```python
from build123d import *

# Parameters (mm, degrees)
F0_W        = 47.8297565132
F0_H        = 76.5759237111
F1_DEPTH    = 40
F2_T1_DEPTH = 274.1378594542
F3_T        = -2


# Not quite as in the source:
# - a fillet or chamfer that OpenCascade refuses, or shapes differently, is made with other operations: its cross-section is extruded or revolved along the edge and cut away or added


with BuildPart() as f1:
    # F0 (on Top) → F1 (new body)
    with BuildSketch(Plane.XY):
        with Locations((-40.5828235671, -10.7496175915)):
            Rectangle(F0_W, F0_H)
    extrude(amount=F1_DEPTH)

    # F2: chamfer of 44 on 1 edges, made by hand

    # F2_s2 → F2_t1 (cut)
    with BuildSketch(Plane.YZ.offset(-177.6517532942)):
        Polygon((27.538344264, -4), (-16.461655736, 40), (27.538344264, 40), align=None)
    extrude(amount=F2_T1_DEPTH, mode=Mode.SUBTRACT)

    # F3
    f3_openings = [f1.faces().sort_by_distance(p)[0] for p in [
        (-40.582824, 3.538344, 20),
    ]]
    offset(amount=F3_T, openings=f3_openings, kind=Kind.INTERSECTION)


solid = f1.part
```
The model under review builds one solid part; all positions refer to its coordinate system, in mm. A direction names the side the tool comes from. Coordinates: 2 decimals unless noted, no trailing zeros. Write each loop counter-clockwise with the first axis right and the second up, starting at its lowest first coordinate (ties: lowest second). Pieces come first, ordered by that corner, then holes. Notation, with made-up numbers: (-20, -25.75) - (-14, -25.75) arc R18 cw to (-14, -20.75) - close; hole circle Ø11 at (76, -25). An arc over 180 degrees is marked (long way). Answer in a Markdown table with one row per item. Add a question column.
Q1. Draft analysis for pull direction X (two halves, no side actions). For faces 3 (the face through (-16.668, -21, 15)), 4 (the face through (-41, -12, 2)), 5 (the face through (-41, -33, 40)), state which applies: +X half, -X half, draft (parallel to the pull), parting line (faces both ways), or undercut.
Q2. To check wall thickness, follow line 1 along X through (y, z) = (-32, 35); line 2 along Z through (x, y) = (-33, -34); line 3 along Y through (x, z) = (-39, 22.5). State the ranges of each line that lie inside material, in increasing order. Write a range as from..to.
Q3. Consider section B-B on y = 2. Give the boundary of the cut face in (x, z).
Q4. For faces 1 (the face through (-41, -47.038, 20)), 2 (the face through (-41, -49.038, 20)), list the 3-axis set-ups (+Z, -Z, +X, -X, +Y, -Y) from which the entire face can be reached by the end or side of a thin tool; tool diameter is ignored.
Q5. Clearance check with flat-ended pins moving along their axes: pin 1 (3 mm diameter, centred on x = -31, y = -7, fed in from +Z); pin 2 (6 mm diameter, centred on x = -31, z = 30, fed in from +Y); pin 3 (4 mm diameter, centred on x = -52, y = -14, fed in from +Z). State where each tip first meets the part, or that it passes through.
Q6. Consider section A-A on y = -30. Give the boundary of the cut face in (x, z).
Q7. Consider section C-C on x = -48. Give the boundary of the cut face in (y, z), then the cut area to 3 significant figures.
Answers below:
| question | item | result |
|---|---|---|
| 1 | face 3 | +X half |
| 1 | face 4 | undercut |
| 1 | face 5 | draft |
| 2 | line 1 | -64.5..-62.5, -18.67..-16.67 |
| 2 | line 2 | 0..2, 38..40 |
| 2 | line 3 | -49.04..-47.04 |
| 3 | outline | (-64.5, 0) - (-16.67, 0) - (-16.67, 21.54) - (-18.67, 21.54) - (-18.67, 2) - (-62.5, 2) - (-62.5, 21.54) - (-64.5, 21.54) - close |
| 4 | face 1 | +Y |
| 4 | face 2 | +Z, -Z, +X, -X, -Y |
| 5 | pin 1 | z = 2 |
| 5 | pin 2 | y = -47.04 |
| 5 | pin 3 | z = 39.54 |
| 6 | outline | (-64.5, 0) - (-16.67, 0) - (-16.67, 40) - (-64.5, 40) - close; hole (-62.5, 2) - (-18.67, 2) - (-18.67, 38) - (-62.5, 38) - close |
| 7 | outline | (-49.04, 0) - (23.54, 0) - (21.54, 2) - (-47.04, 2) - (-47.04, 38) - (-14.46, 38) - (-16.46, 40) - (-49.04, 40) - close |
| 7 | area | 282 mm² |
